```python
from build123d import *

# Parameters (mm, degrees)
SKETCH1_W           = 55
SKETCH1_H           = 55
SKETCH1_R           = 1.75
BOSS_EXTRUDE1_DEPTH = 3
SKETCH2_W           = 22.5
SKETCH2_H           = 22.5
SKETCH2_W_2         = 16.5
SKETCH2_H_2         = 16.5
BOSS_EXTRUDE2_DEPTH = 30
SKETCH3_W           = 16.5
SKETCH3_H           = 16.5
CUT_EXTRUDE1_DEPTH  = 30
FILLET1_R           = 4
FILLET2_R           = 4


with BuildPart() as part:
    # Sketch1 → Boss-Extrude1 (new body)
    with BuildSketch(Plane(origin=(0, 0, 0), x_dir=(1, 0, 0), z_dir=(0, 1, 0))):
        Rectangle(SKETCH1_W, SKETCH1_H)
        with Locations(Location((20.140368527, 20.140368527, 0), (0, 0, 270))):
            Circle(SKETCH1_R, mode=Mode.SUBTRACT)
        with Locations(Location((-19.859631473, -19.859631473, 0), (0, 0, 270))):
            Circle(SKETCH1_R, mode=Mode.SUBTRACT)
        with Locations(Location((-20.140368527, 20.140368527, 0), (0, 0, 90))):
            Circle(SKETCH1_R, mode=Mode.SUBTRACT)
        with Locations(Location((19.859631473, -19.859631473, 0), (0, 0, 90))):
            Circle(SKETCH1_R, mode=Mode.SUBTRACT)
    extrude(amount=BOSS_EXTRUDE1_DEPTH)

    # Sketch2 → Boss-Extrude2 (add)
    with BuildSketch(Plane(origin=(0, 3, 0), x_dir=(1, 0, 0), z_dir=(0, 1, 0))):
        Rectangle(SKETCH2_W, SKETCH2_H)
        Rectangle(SKETCH2_W_2, SKETCH2_H_2, mode=Mode.SUBTRACT)
    extrude(amount=BOSS_EXTRUDE2_DEPTH)

    # Sketch3 → Cut-Extrude1 (cut)
    with BuildSketch(Plane(origin=(0, 3, 0), x_dir=(1, 0, 0), z_dir=(0, 1, 0))):
        Rectangle(SKETCH3_W, SKETCH3_H)
    extrude(amount=-CUT_EXTRUDE1_DEPTH, mode=Mode.SUBTRACT)

    # Fillet1
    fillet1_edges = [part.edges().sort_by_distance(p)[0] for p in [
        (-11.25, 3, 0),
        (0, 3, 11.25),
        (11.25, 3, 0),
        (0, 3, -11.25),
    ]]
    fillet(fillet1_edges, radius=FILLET1_R)

    # Fillet2
    fillet2_edges = [part.edges().sort_by_distance(p)[0] for p in [
        (27.5, 1.5, 27.5),
        (-27.5, 1.5, 27.5),
        (-27.5, 1.5, -27.5),
        (27.5, 1.5, -27.5),
    ]]
    fillet(fillet2_edges, radius=FILLET2_R)


solid = part.part
```
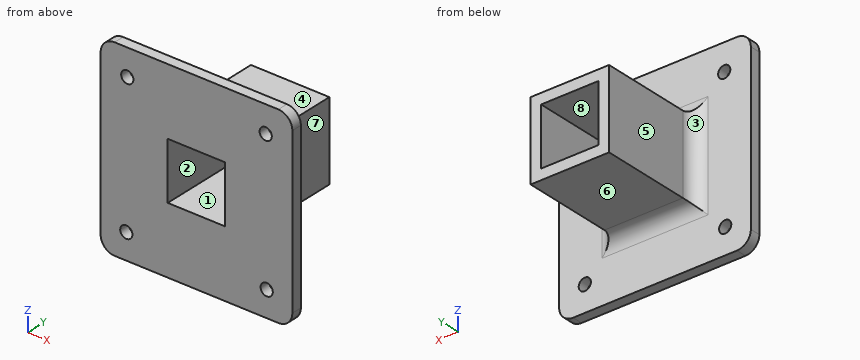
Could you check a few things on this model? Use its own coordinates, in mm. Face numbers are marked on the shaded views. A direction names the side the tool comes from. Round coordinates to 2 decimals unless told otherwise and drop trailing zeros. Loops run counter-clockwise (first coordinate to the right, second up) from the corner with the lowest first, then second, coordinate; pieces in that order, holes last.
Q1. For P1, Ø2, axis at x = -5.5, y = 5.5, coming from the +Z side; P2, Ø7, axis at y = 19.5, z = -0.5, coming from the +X side; P3, Ø16.5, axis at x = -5.5, z = 1, coming from the +Y side; P4, Ø11, axis at y = 20, z = 5, coming from the -X side, each with a flat end and sliding along its axis, tell me the tip position at first contact or that it passes through.
Q2. I want a section at A-A (x = 4). Write out the boundary of the cut face in (y, z), and give its area (3 significant figures).
Q3. On a 3-axis mill with a long thin cutter (end or side, diameter ignored), from which of +Z, -Z, +X, -X, +Y, -Y can I reach the whole of each face in a straight line? I mean the marked faces 5, 6, 7 and 8. Say none if no direction works.
Q4. I want a section at C-C (z = 4.5). Write out the boundary of the cut face in (x, y), and give its area (3 significant figures).
Q5. Thinking about a two-plate mould opening in Z: for the marked faces 1, 2, 3 and 4, which applies, pulls with the +Z half, pulls with the -Z half, needs draft (parallel to the pull), parting line crosses it, or undercut?
Q6. I want a section at D-D (z = -19.5). Write out the boundary of the cut face in (x, y), and give its area (3 significant figures).
Q7. I want a section at B-B (y = 31). Write out the boundary of the cut face in (x, z), and give its area (3 significant figures).
Q8. Please list where these lines run through material, in increasing order: L1, parallel to X at y = 13.5, z = -2.5; L2, parallel to Y at x = 20, z = -11.5.
Answer below:
1. P1: stops at z = 12.13
1. P2: stops at x = 11.25
1. P3: stops at y = 33
1. P4: stops at x = -11.25
2. outline: (0, -27.5) - (3, -27.5) - (3, -15.25) arc R4 cw to (7, -11.25) - (33, -11.25) - (33, -8.25) - (0, -8.25) - close; (0, 8.25) - (33, 8.25) - (33, 11.25) - (7, 11.25) arc R4 cw to (3, 15.25) - (3, 27.5) - (0, 27.5) - close
2. area: 302 mm2
3. face 5: +Z, -Z, -X, +Y
3. face 6: -Z, +X, -X, +Y
3. face 7: +Z, -Z, +X, +Y
3. face 8: +Y, -Y
4. outline: (-27.5, 0) - (-8.25, 0) - (-8.25, 33) - (-11.25, 33) - (-11.25, 7) arc R4 cw to (-15.25, 3) - (-27.5, 3) - close; (8.25, 0) - (27.5, 0) - (27.5, 3) - (15.25, 3) arc R4 cw to (11.25, 7) - (11.25, 33) - (8.25, 33) - close
4. area: 302 mm2
5. face 1: undercut
5. face 2: undercut
5. face 3: needs draft
5. face 4: pulls with the +Z half
6. outline: (-27.5, 0) - (-21.77, 0) - (-21.77, 3) - (-27.5, 3) - close; (-18.51, 0) - (18.51, 0) - (18.51, 3) - (-18.51, 3) - close; (21.77, 0) - (27.5, 0) - (27.5, 3) - (21.77, 3) - close
6. area: 145 mm2
7. outline: (-11.25, -11.25) - (11.25, -11.25) - (11.25, 11.25) - (-11.25, 11.25) - close; hole (-8.25, -8.25) - (8.25, -8.25) - (8.25, 8.25) - (-8.25, 8.25) - close
7. area: 234 mm2
8. L1: x = -11.25 to -8.25, 8.25 to 11.25
8. L2: y = 0 to 3
